Part model, mm, in its own coordinate system. A direction names the side the tool comes from. Round coordinates to 2 decimals unless told otherwise and drop trailing zeros. Write each loop counter-clockwise with the first axis right and the second up, starting at its lowest first coordinate (ties: lowest second). Pieces come first, ordered by that corner, then holes. Notation, with made-up numbers: (38.5, 19) -> (75.5, 19) arc R14 cw to (75.5, 42) -> close; hole circle Ø9 at (20, 45). An arc over 180 degrees is marked (long way). Return JSON: item names as keys, results as strings. Group by question number.
(1) Saw through at B-B (y = -9.25). List the corners of the cut face in (x, z), plus the area to 3 significant figures.
(2) Tool access for faces 4 (the flat face through (283.573, -13, -60)), 5 (the flat face through (246, -12, -2.54)), 6 (the flat face through (213.36, -13, 55)): list every direction of +Z, -Z, +X, -X, +Y, -Y with a clear straight run to the whole face (end or side of a thin tool).
(3) Saw through at A-A (z = -41). List the corners of the cut face in (x, y).
(4) Saw through at D-D (z = 42). List the corners of the cut face in (x, y), plus the area to 3 significant figures.
(5) Drill centre lines: L1, parallel to Z at x = 105.5, y = -20.5; L2, parallel to X at y = -4.25, z = -1.5; L3, parallel to X at y = -8, z = 41. Where is each one in solid material? Low to high. Write a range as from..to.
(6) Drop flat-ended pins along their axis: pin 1 Ø7.5 at (y, z) = (-16.5, 70) entering from +X; pin 2 Ø10 at (x, z) = (91, 80) entering from +Y. Give the stop position or say it passes through.
(7) Mould opens along Z. For faces 1 (the flat face through (281.033, -12, -59)), 2 (the flat face through (140, -13, -118.793)), 3 (the flat face through (0, -13, -5)) say: +Z half, -Z half, draft (parallel to the pull), parting line (faces both ways), or undercut.
(8) Saw through at C-C (x = 56). List the corners of the cut face in (y, z), plus the area to 3 significant figures.
from build123d import *

# Parameters (mm, degrees)
F0_W     = 213.3595049381
F0_H     = 111.76
F1_DEPTH = 25.4
F2_T     = -2.54
F3_W     = 283.5729122162
F3_H     = 118.7930554152
F4_DEPTH = 25.4
F5_T     = -2.54


# Not quite as in the source:
# - a shell that OpenCascade refuses in one call is made with other operations: the cavity is built on its own and cut out


with BuildPart() as f1:
    # F0 (on Front) → F1 (new body)
    with BuildSketch(Plane.XZ):
        with Locations((106.6797524691, 55.88)):
            Rectangle(F0_W, F0_H)
    extrude(amount=F1_DEPTH)

    # F2
    f2_openings = [f1.faces().sort_by_distance(p)[0] for p in [
        (106.679752, 0, 55.88),
    ]]
    offset(amount=F2_T, openings=f2_openings)

    # F3 (on Front) → F4 (join)
    with BuildSketch(Plane.XZ):
        with Locations((141.7864561081, -59.3965277076)):
            Rectangle(F3_W, F3_H)
    extrude(amount=F4_DEPTH)

    # F5: a shell. OpenCascade refuses it in one call, so the cavity is built on its own and cut out:
    # the body offset inwards by the wall thickness, plus a prism from it out through each open face.
    f5_core = offset(f1.part, amount=F5_T, kind=Kind.INTERSECTION, mode=Mode.PRIVATE)
    f5_exits = [f5_core.faces().sort_by_distance(p)[0] for p in [
        (141.209622, -2.54, -58.441458),
    ]]
    add(f5_core, mode=Mode.SUBTRACT)
    extrude(f5_exits, amount=-F5_T, mode=Mode.SUBTRACT)


solid = f1.part
Computed values:
{
 "1": {"outline": "(0, -118.79) -> (283.57, -118.79) -> (283.57, 0) -> (213.36, 0) -> (213.36, 111.76) -> (0, 111.76) -> close; hole (2.54, -116.25) -> (281.03, -116.25) -> (281.03, -2.54) -> (210.82, -2.54) -> (210.82, 0) -> (2.54, 0) -> close; hole (2.54, 2.54) -> (210.82, 2.54) -> (210.82, 109.22) -> (2.54, 109.22) -> close", "area": "3,110 mm2"},
 "2": {"face 4": "+Z, -Z, +X, +Y, -Y", "face 5": "+Y", "face 6": "+Z, +X, +Y, -Y"},
 "3": {"outline": "(0, -25.4) -> (283.57, -25.4) -> (283.57, 0) -> (281.03, 0) -> (281.03, -22.86) -> (2.54, -22.86) -> (2.54, 0) -> (0, 0) -> close"},
 "4": {"outline": "(0, -25.4) -> (213.36, -25.4) -> (213.36, 0) -> (210.82, 0) -> (210.82, -22.86) -> (2.54, -22.86) -> (2.54, 0) -> (0, 0) -> close", "area": "658 mm2"},
 "5": {"L1": "-118.79..-116.25, 0..2.54, 109.22..111.76", "L2": "0..2.54, 210.82..283.57", "L3": "0..2.54, 210.82..213.36"},
 "6": {"pin 1": "x = 213.36", "pin 2": "y = -22.86"},
 "7": {"face 1": "undercut", "face 2": "-Z half", "face 3": "draft"},
 "8": {"outline": "(-25.4, -118.79) -> (0, -118.79) -> (0, -116.25) -> (-22.86, -116.25) -> (-22.86, 0) -> (0, 0) -> (0, 2.54) -> (-22.86, 2.54) -> (-22.86, 109.22) -> (0, 109.22) -> (0, 111.76) -> (-25.4, 111.76) -> close", "area": "760 mm2"}
}
